```python
from build123d import *

# Parameters (mm, degrees)
CYLINDER001_R        = 0.625
CYLINDER001_DEPTH    = 10
CYLINDER002_R        = 2
CYLINDER002_DEPTH    = 76.2
CYLINDER_R           = 0.625
CYLINDER_DEPTH       = 13.75
CYLINDER_PITCH_ANGLE = -90


with BuildPart() as cylinder001:
    # Cylinder001 → Cylinder001 (new body)
    with BuildSketch(Plane.XY):
        Circle(CYLINDER001_R)
    extrude(amount=CYLINDER001_DEPTH)


with BuildPart() as cylinder002:
    # Cylinder002 → Cylinder002 (new body)
    with BuildSketch(Plane.XY.offset(30)):
        Circle(CYLINDER002_R)
    extrude(amount=CYLINDER002_DEPTH)


with BuildPart() as cone:
    # Cone → Cone (revolve)
    with BuildSketch(Plane(origin=(0, 0, 10), x_dir=(1, 0, 0), z_dir=(0, -1, 0))):
        Polygon((0, 0), (0.625, 0), (2, 20), (0, 20), align=None)
    revolve(axis=Axis((0, 0, 10), (0, 0, 1)))


with BuildPart() as sphere001:
    # Sphere001 → Sphere001 (revolve)
    with BuildSketch(Plane(origin=(7.5, 0, 0), x_dir=(1, 0, 0), z_dir=(0, -1, 0))):
        with BuildLine():
            ThreePointArc((0, -1.25), (1.25, 0), (0, 1.25))
            Line((0, 1.25), (0, -1.25))
        make_face()
    revolve(axis=Axis((7.5, 0, 0), (0, 0, 1)))


with BuildPart() as cylinder:
    # Cylinder → Cylinder (new body)
    with BuildSketch(Plane.XY):
        Circle(CYLINDER_R)
    extrude(amount=CYLINDER_DEPTH)


with BuildPart() as cylinder_1:
    # Cylinder pitch: moved
    add(cylinder.part.rotate(Axis((0, 0, 0), (0, 1, 0)), CYLINDER_PITCH_ANGLE))


with BuildPart() as cylinder_2:
    # Cylinder placement: moved
    add(cylinder_1.part.moved(Location((6.875, 0, 0))))


with BuildPart() as fusion:
    # Sphere → Sphere (revolve)
    with BuildSketch(Plane(origin=(-6.25, 0, 0), x_dir=(1, 0, 0), z_dir=(0, -1, 0))):
        with BuildLine():
            ThreePointArc((0, -2.5), (2.5, 0), (0, 2.5))
            Line((0, 2.5), (0, -2.5))
        make_face()
    revolve(axis=Axis((-6.25, 0, 0), (0, 0, 1)))

    # Fusion: union Cylinder001, Cylinder002, Cone, Sphere001, Cylinder
    add(cylinder001.part)
    add(cylinder002.part)
    add(cone.part)
    add(sphere001.part)
    add(cylinder_2.part)


solid = fusion.part
```
Can you work these out from the model? Positions are in its coordinate system, mm. Give positions to 0.01 mm unless a question says otherwise; leave off trailing zeros. Loops run counter-clockwise (first coordinate to the right, second up) from the corner with the lowest first, then second, coordinate; pieces in that order, holes last. Notation, with made-up numbers: M 82,49 L 96,49 A38 ccw 96,87 Z; hole C 38.25,-16.5 d9. An arc over 180 degrees is marked long. One line per question, with ' | ' between items. Start each with the question number.
Q1. If we mould it in two halves opening along Z, with no side actions, what happens to faces 1 (the flat face through (0, 0, 106.2)), 2 (the cylindrical face through (0, -2, 68)), 3 (the conical face through (-0.17, 1.31, 20.14))? For each: +Z half, -Z half, draft (parallel to the pull), parting line (faces both ways), or undercut.
Q2. If we section it at A-A (z = 46): Please give me the cut outline in (x, y), plus the area to 3 significant figures.
Q3. If I drill on line 1 (X direction, y = -1.55, z = 81); line 2 (X direction, y = -0.05, z = 42.5); line 3 (Y direction, x = -1, z = 95.5), over which ranges is the centre line in solid material (lowest first)? Write a range as from..to.
Q4. For pin 1 Ø6 at (x, z) = (-7, 89) entering from +Y; pin 2 Ø3 at (x, y) = (1.5, -0.5) entering from -Z (3 decimals); pin 3 Ø1.5 at (x, y) = (-1.5, 2) entering from +Z, each with a flat end and sliding along its axis, tell me the tip position at first contact or that it passes through.
Q5. If we section it at B-B (x = -7.5): Please give me the cut outline in (y, z).
Computed:
1) face 1: +Z half | face 2: draft | face 3: undercut
2) outline: C 0,0 d4 | area: 12.6 mm²
3) line 1: x = -1.26..1.26 | line 2: x = -2..2 | line 3: y = -1.73..1.73
4) pin 1: passes through | pin 2: stops at z = -0.625 | pin 3: stops at z = 106.2
5) outline: C 0,0 d4.33
